Source: CAD feature listing. Evaluate the final solid. Frame: model axes, mm. Face numbers are marked on the shaded views. A direction names the side the tool comes from. Coordinates: 2 decimals unless noted, no trailing zeros. Loops run counter-clockwise (first coordinate to the right, second up) from the corner with the lowest first, then second, coordinate; pieces in that order, holes last.
Item 1: Section query D-D, the plane x = -6.25. Return the cut outline in (y, z), then the cut area to 3 significant figures.
Item 2: Section query C-C, the plane x = 1.75. Return the cut outline in (y, z).
Item 3: Pin query (flat end, axial travel): pin 1 Ø2 at (x, y) = (-8.5, 0) entering from +Z; pin 2 Ø3 at (x, z) = (-12.5, -4.5) entering from -Y; pin 3 Ø3 at (x, y) = (-7.5, 5) entering from -Z. Return the tip coordinate at first contact, or that it passes through.
Item 4: Reachability of the marked faces 1 and 2 from +Z, -Z, +X, -X, +Y, -Y: full face, straight path, thin tool, end or side. Return the list, or none.
Item 5: Section query A-A, the plane z = 0. Return the cut outline in (x, y).
Item 6: Line query: probe 1 along X at (y, z) = (-4.5, -2.25); probe 2 along Z at (x, y) = (-16.25, 0.75); probe 3 along X at (y, z) = (5, -2.25). Output: solid intervals per line, ascending.
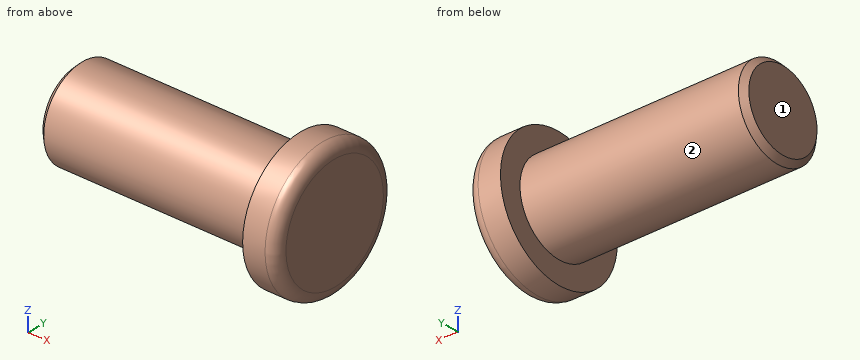
```python
from build123d import *

# Parameters (mm, degrees)
SKETCH1_R           = 6
SKETCH1_R_2         = 4
BOSS_EXTRUDE1_DEPTH = 3
BOSS_EXTRUDE2_START = -23
SKETCH2_R           = 4
BOSS_EXTRUDE2_DEPTH = 23
FILLET1_R           = 1
CHAMFER1_SIZE       = 0.5


with BuildPart() as part:
    # Sketch1 → Boss-Extrude1 (new body)
    with BuildSketch(Plane(origin=(0, 0, 0), x_dir=(0, 0, -1), z_dir=(1, 0, 0))):
        Circle(SKETCH1_R)
        Circle(SKETCH1_R_2, mode=Mode.SUBTRACT)
    extrude(amount=BOSS_EXTRUDE1_DEPTH)

    # Sketch2 → Boss-Extrude2 (add)
    with BuildSketch(Plane(origin=(3, 0, 0), x_dir=(0, 0, -1), z_dir=(1, 0, 0)).offset(BOSS_EXTRUDE2_START)):
        Circle(SKETCH2_R)
    extrude(amount=BOSS_EXTRUDE2_DEPTH)

    # Fillet1
    fillet1_edges = [part.edges().sort_by_distance(p)[0] for p in [
        (3, 0, 6),
    ]]
    fillet(fillet1_edges, radius=FILLET1_R)

    # Chamfer1
    chamfer1_edges = [part.edges().sort_by_distance(p)[0] for p in [
        (-20, 0, 4),
    ]]
    chamfer(chamfer1_edges, length=CHAMFER1_SIZE)


solid = part.part
```
Verdict:
1. outline: circle Ø8 at (0, 0)
1. area: 50.3 mm2
2. outline: circle Ø12 at (0, 0)
3. pin 1: stops at z = 4
3. pin 2: stops at y = -2.65
3. pin 3: stops at z = -1.94
4. face 1: +Z, -Z, -X, +Y, -Y
4. face 2: -X
5. outline: (-20, -3.5) - (-19.5, -4) - (0, -4) - (0, -6) - (2, -6) arc R1 ccw to (3, -5) - (3, 5) arc R1 ccw to (2, 6) - (0, 6) - (0, 4) - (-19.5, 4) - (-20, 3.5) - close
6. probe 1: x = 0 to 3
6. probe 2: z = -3.93 to 3.93
6. probe 3: x = 0 to 2.88
